Part print with two shaded views. Sizes in mm from the minimum x, y, z corner. A direction names the side the tool comes from. Round coordinates to 2 decimals unless told otherwise and drop trailing zeros. Write each loop counter-clockwise with the first axis right and the second up, starting at its lowest first coordinate (ties: lowest second). Pieces come first, ordered by that corner, then holes. Notation, with made-up numbers: M 24,-11 L 65,-11 A20 cw 65,17 Z; hole C 82.25,16 d1. An arc over 180 degrees is marked long. Use one line per item in the form item = value. Start each with the question number.
Item 1: Flat gauge pins, fed straight in: pin 1 Ø4 at (y, z) = (3, 2.5) entering from +X; pin 2 Ø5 at (y, z) = (7.5, 4) entering from -X; pin 3 Ø4.5 at (x, z) = (39.5, 5) entering from -Y. Where does each tip first touch, or does it go through?
Item 2: Cut at D-D, the plane z = 2.5. Give the cut face in (x, y), then the cut area to 3 significant figures.
Item 3: Cut at B-B, the plane z = 5. Give the cut face in (x, y), then the cut area to 3 significant figures.
Item 4: Which spindle directions (+Z, -Z, +X, -X, +Y, -Y) get a long thin tool onto all of the face, cutting with end or side? Do the marked faces 1, 2 and 3. Say none if no direction does.
Item 5: Cut at C-C, the plane y = 18.5. Give the cut face in (x, z).
Item 6: Cut at A-A, the plane x = 39.5. Give the cut face in (y, z), then the cut area to 3 significant figures.
Item 7: Probe L1, parallel to Z at x = 39.5, y = 19.3; L2, parallel to Y at x = 9.5, z = 9.25; L3, parallel to X at y = 8.5, z = 2.25. List the from-to ranges inside material, lowest first.
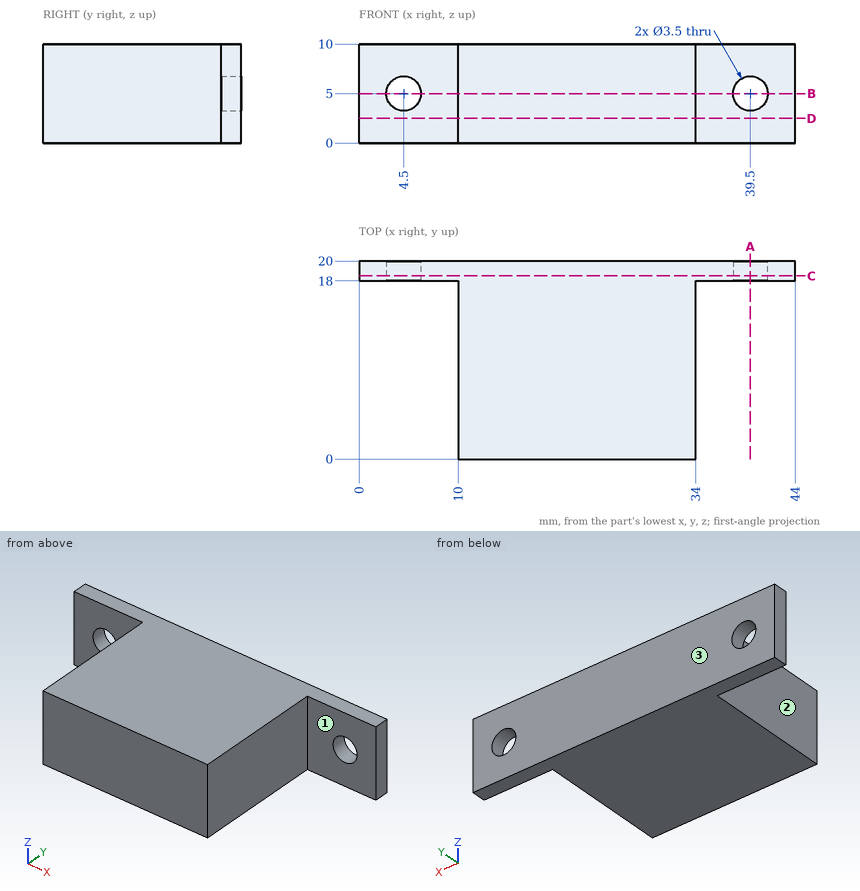
Model answer:
q1.pin_1 = 34
q1.pin_2 = 10
q1.pin_3 = 18
q2.outline = M 0,18 L 10,18 L 10,0 L 34,0 L 34,18 L 44,18 L 44,20 L 0,20 Z
q2.area = 520 mm²
q3.outline = M 0,18 L 2.75,18 L 2.75,20 L 0,20 Z; M 6.25,18 L 10,18 L 10,0 L 34,0 L 34,18 L 37.75,18 L 37.75,20 L 6.25,20 Z; M 41.25,18 L 44,18 L 44,20 L 41.25,20 Z
q3.area = 506 mm²
q4.face_1 = +Z, -Z, +X, -Y
q4.face_2 = +Z, -Z, -X, -Y
q4.face_3 = +Z, -Z, +X, -X, +Y
q5.outline = M 0,0 L 44,0 L 44,10 L 0,10 Z; hole C 4.5,5 d3.5; hole C 39.5,5 d3.5
q6.outline = M 18,0 L 20,0 L 20,3.25 L 18,3.25 Z; M 18,6.75 L 20,6.75 L 20,10 L 18,10 Z
q6.area = 13.0 mm²
q7.L1 = 0 to 3.25, 6.75 to 10
q7.L2 = 18 to 20
q7.L3 = 10 to 34
